Geometry check sheet. Reference: the model listing, model coordinates, mm. Face numbers are marked on the shaded views. A direction names the side the tool comes from. Give positions to 0.01 mm unless a question says otherwise; leave off trailing zeros. Write each loop counter-clockwise with the first axis right and the second up, starting at its lowest first coordinate (ties: lowest second). Pieces come first, ordered by that corner, then holes.
(1) Depth check by flat-ended pin: P1, Ø8, axis at x = -18, z = 26.5, coming from the -Y side; P2, Ø3, axis at x = 20.5, z = 26, coming from the -Y side; P3, Ø1.5, axis at y = 18, z = 35.5, coming from the +X side. Enter the tip coordinate at first touch or a pass-through.
(2) Cross-section at D-D (z = 40). Record the boundary of the cut face in (x, y), and give its area (3 significant figures).
(3) Thickness scan on line 1 along Z through (x, y) = (108, 19); line 2 along Y through (x, z) = (140.5, 36); line 3 along X through (y, z) = (4.5, 46). Record the ranges inside material, lowest first.
(4) Mould release check, pull along Z, two halves, no side actions. Record for the marked faces 1, 2 and 3: +Z half, -Z half, draft (parallel to the pull), parting line (faces both ways), or undercut.
(5) Cross-section at B-B (z = 28.5). Record the boundary of the cut face in (x, y), and give its area (3 significant figures).
(6) Cross-section at A-A (x = 108). Record the boundary of the cut face in (y, z), and give its area (3 significant figures).
(7) Tool access check on the marked faces 4 and 5. Record the directions out of +Z, -Z, +X, -X, +Y, -Y that give a thin tool (end or side, any length) a straight path to the whole face; none if there is none.
(8) Cross-section at C-C (y = 18.5). Count the separate pieces of the cut face and the enclosed holes in it, and give its area (3 significant figures).
```python
from build123d import *

# Parameters (mm, degrees)
F1_DEPTH = 52
F4_R     = 11
F5_DEPTH = 38
F6_R     = 25.99999


# Not quite as in the source:
# - a fillet or chamfer is up to 0.001 mm smaller than in the source, because OpenCascade refuses the exact size


with BuildPart() as f1:
    # F0 (on Top) → F1 (new body)
    with BuildSketch(Plane.XY):
        with BuildLine():
            Line((182, 38), (61.1555394057, 38))
            ThreePointArc((61.1555394057, 38), (-19.7585571689, 69.2358246763), (-72, 0))
            Line((-72, 0), (182, 0))
            Line((182, 0), (182, 38))
        make_face()
    extrude(amount=F1_DEPTH)

    # F2 (on face) → F3 (revolve, cut)
    with BuildSketch(Plane.XZ):
        Polygon((60, 52), (0, 52), (0, 0), (42, 0), align=None)
    revolve(axis=Axis((0, 0, 26), (0, 0, -1)), mode=Mode.SUBTRACT)

    # F4 (on face) → F5 (cut)
    with BuildSketch(Plane.XZ):
        with Locations((108, 25.7937852293)):
            Circle(F4_R)
        with Locations((156, 25.2048280338)):
            Circle(F4_R)
    extrude(amount=-F5_DEPTH, mode=Mode.SUBTRACT)

    # F6 (radius 26 in the source; OpenCascade refuses exactly that, so slightly less here)
    f6_edges = [f1.edges().sort_by_distance(p)[0] for p in [
        (182, 19, 52),
        (182, 19, 0),
    ]]
    fillet(f6_edges, radius=F6_R)


solid = f1.part
```
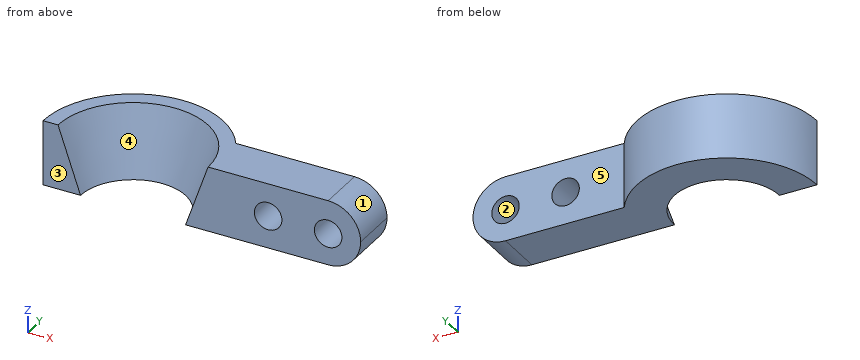
Reply:
1. P1: stops at y = 45.66
1. P2: stops at y = 45.81
1. P3: stops at x = 180.48
2. outline: (-72, 0) - (-55.85, 0) arc R55.85 cw to (55.85, 0) - (177.91, 0) - (177.91, 38) - (61.16, 38) arc R72 ccw to start
2. area: 7,400 mm2
3. line 1: z = 0 to 14.79, 36.79 to 52
3. line 2: y = 0 to 38
3. line 3: x = -71.86 to -57.75, 57.75 to 172.61
4. face 1: +Z half
4. face 2: undercut
4. face 3: draft
5. outline: (-72, 0) - (-51.87, 0) arc R51.87 cw to (51.87, 0) - (97.34, 0) - (97.34, 38) - (61.16, 38) arc R72 ccw to start; (118.66, 0) - (145.51, 0) - (145.51, 38) - (118.66, 38) - close; (166.49, 0) - (181.88, 0) - (181.88, 38) - (166.49, 38) - close
5. area: 6,620 mm2
6. outline: (0, 0) - (38, 0) - (38, 14.79) - (0, 14.79) - close; (0, 36.79) - (38, 36.79) - (38, 52) - (0, 52) - close
6. area: 1,140 mm2
7. face 4: +Z, -Y
7. face 5: +Z, -Z, +X, +Y
8. separate pieces: 2
8. enclosed holes: 2
8. area: 7,090 mm2
